from build123d import *

# Parameters (mm, degrees)
BOSS_EXTRU_1_DEPTH      = 7
ESQUISSE2_R             = 1.4
ENL_V_MAT_EXTRU_1_DEPTH = 16.13274595
ESQUISSE3_R             = 0.95
ENL_V_MAT_EXTRU_2_DEPTH = 10
CONG_1_R                = 4
CONG_2_R                = 3
CONG_3_R                = 3.5
CONG_4_R                = 5


with BuildPart() as part:
    # Esquisse1 → Boss.-Extru.1 (new body)
    with BuildSketch(Plane.XY):
        Polygon((-2, 13), (0, 9), (0, 3), (-6, 3), (-6, 0), (0, 0), (6, 0), (6, 15), (-2, 15), align=None)
    extrude(amount=BOSS_EXTRU_1_DEPTH)

    # Esquisse2 → Enlèv. mat.-Extru.1 (cut, through all)
    with BuildSketch(Plane(origin=(0, 3, 0), x_dir=(1, 0, 0), z_dir=(0, 1, 0))):
        with Locations(Location((-3, -4, 0), (0, 0, 180))):
            Circle(ESQUISSE2_R)
    extrude(amount=-ENL_V_MAT_EXTRU_1_DEPTH, mode=Mode.SUBTRACT)

    # Esquisse3 → Enlèv. mat.-Extru.2 (cut)
    with BuildSketch(Plane(origin=(0, 15, 0), x_dir=(1, 0, 0), z_dir=(0, 1, 0))):
        with Locations(Location((3, -3.5, 0), (0, 0, 270))):
            Circle(ESQUISSE3_R)
    extrude(amount=-ENL_V_MAT_EXTRU_2_DEPTH, mode=Mode.SUBTRACT)

    # Congé1
    cong_1_edges = [part.edges().sort_by_distance(p)[0] for p in [
        (-6, 1.5, 0),
    ]]
    fillet(cong_1_edges, radius=CONG_1_R)

    # Congé2
    cong_2_edges = [part.edges().sort_by_distance(p)[0] for p in [
        (-6, 1.5, 7),
    ]]
    fillet(cong_2_edges, radius=CONG_2_R - 0.0001)  # a hair under: the kernel refuses the full size

    # Congé3
    cong_3_edges = [part.edges().sort_by_distance(p)[0] for p in [
        (6, 7.5, 7),
        (6, 7.5, 0),
    ]]
    fillet(cong_3_edges, radius=CONG_3_R - 0.0001)  # a hair under: the kernel refuses the full size

    # Congé4
    cong_4_edges = [part.edges().sort_by_distance(p)[0] for p in [
        (0, 9, 3.5),
        (-2, 13, 3.5),
    ]]
    fillet(cong_4_edges, radius=CONG_4_R)


solid = part.part
CAD build for the part. Positions are in the model's coordinates, mm. A direction names the side the tool comes from. Round coordinates to 2 decimals unless told otherwise and drop trailing zeros. Write each loop counter-clockwise with the first axis right and the second up, starting at its lowest first coordinate (ties: lowest second). Pieces come first, ordered by that corner, then holes. Notation, with made-up numbers: M 70,85 L 90,85 A29 ccw 90,115 Z; hole C 43.5,54.25 d1. An arc over 180 degrees is marked long. Put each result on its own line as item: value. Start each with the question number.
1) Drill centre lines: probe 1 along Z at (x, y) = (2.75, 6.5); probe 2 along Y at (x, z) = (-3.25, 1.5); probe 3 along X at (y, z) = (12, 3.5). Where is each one in solid material? Low to high. Write a range as [from, to].
2) Saw through at C-C, the plane z = 6.5. Write the cut outline in (x, y).
3) Pull direction X, two halves, no side cores. Call faces 1 (the cylindrical face through (3.64, 10.07, 2.8)), 2 (the cylindrical face through (4.95, 7.6, 6)), 3 (the cylindrical face through (-1.87, 13.05, 3.55)): pulls with the +X half, pulls with the -X half, needs draft (parallel to the pull), parting line crosses it, or undercut.
4) Saw through at D-D, the plane x = 3. Write the cut outline in (y, z).
5) 3-axis set-ups, long thin cutter, end or side, ignore diameter. For faces 4 (the flat face through (-2, 14.6, 3.5)), 5 (the cylindrical face through (-0.13, 8.95, 3.55)), 6 (the flat face through (3, 5, 3)), 7 (the cylindrical face through (-2.697, 1.521, 2.633)): which of +Z, -Z, +X, -X, +Y, -Y reach the whole face in a straight line?
6) Pin check, flat tips, straight feed: pin 1 Ø0.7 at (y, z) = (14.5, 5) entering from -X; pin 2 Ø0.6 at (x, z) = (3.5, 3.5) entering from +Y; pin 3 Ø2 at (x, y) = (-4, 3.5) entering from -Z. Stop position of each tip, or through.
7) Saw through at A-A, the plane x = -0.75. Write the cut outline in (y, z).
Resolved:
1. probe 1: [0.01, 2.58], [4.42, 6.99]
1. probe 2: [0, 3]
1. probe 3: [-1.5, 2.05], [3.95, 6]
2. outline: M -4.66,0 L 4.3,0 L 4.3,15 L -2,15 L -2,14.18 A5 ccw -1.47,11.94 L -0.53,10.06 A5 cw 0,7.82 L 0,3 L -4.66,3 Z
3. face 1: undercut
3. face 2: pulls with the +X half
3. face 3: pulls with the -X half
4. outline: M 0,0.04 L 15,0.04 L 15,2.55 L 5,2.55 L 5,4.45 L 15,4.45 L 15,6.96 L 0,6.96 Z
5. face 4: +Z, -Z, -X, +Y
5. face 5: +Z, -Z, -X
5. face 6: +Y
5. face 7: -Y
6. pin 1: x = -2
6. pin 2: y = 5
6. pin 3: z = 0.16
7. outline: M 0,0 L 3,0 L 3,7 L 0,7 Z; M 10.5,0 L 15,0 L 15,7 L 10.5,7 Z
